Input: part model. Units: mm. Frame: model coordinates. A direction names the side the tool comes from. Round coordinates to 2 decimals unless told otherwise and drop trailing zeros. Loops run counter-clockwise (first coordinate to the right, second up) from the corner with the lowest first, then second, coordinate; pieces in that order, holes last.
1) Section A-A, the plane y = 0. Return loops of the section in (x, z).
2) Section C-C, the plane x = 4. Return loops of the section in (y, z), and give its area (3 significant figures).
3) Section B-B, the plane z = -10.5. Return loops of the section in (x, y), and give its area (3 significant figures).
4) First-contact query: pin 1 (4.5 mm diameter, centred on y = -22, z = 0.03, fed in from -X); pin 2 (4 mm diameter, centred on y = -11.03, z = -19.04, fed in from -X); pin 3 (2 mm diameter, centred on y = -1, z = 14.5, fed in from +X). Flat tips, straight axial feed; report the tip coordinate or a pass-through.
5) Access query for faces 5 (the face through (22, 4, 14)), 6 (the face through (32.5, 0, -14)), 7 (the face through (7.5, 15, -7)). Directions: +Z, -Z, +X, -X, +Y, -Y. A direction counts if a zero-diameter tool reaches every point of the face in a straight line with its end or side. Return the directions, or none.
6) Ray query, line 1 along Y through (x, z) = (22, 0.5); line 2 along X through (y, z) = (26, -3); line 3 along Z through (x, y) = (16.5, 22). Return the intervals inside material, ascending.
7) Draft query along Z for faces 1 (the face through (-0.11, 15.5, -4.88)), 2 (the face through (-7.5, 8, -10)), 3 (the face through (21.52, -10.9, -18.63)), 4 (the face through (13.99, 10.92, 16.58)). Return one class per face: pulls with the +Z half, pulls with the -Z half, needs draft (parallel to the pull), parting line crosses it, or undercut.
8) Section D-D, the plane z = 25. Return loops of the section in (x, y), and give its area (3 significant figures).
Autodesk Inventor part; units mm, degrees
ref_plane "YZ Plane" through (0, 0, 0) normal (1, 0, 0) x (0, 1, 0)
ref_plane "XZ Plane" through (0, 0, 0) normal (0, 1, 0) x (-1, 0, 0)
ref_plane "XY Plane" through (0, 0, 0) normal (0, 0, 1) x (1, 0, 0)
sketch "Skizze1" plane through (0, 0, 0) normal (1, 0, 0) x (0, 1, 0)
  circle A0 centre (0, 0) radius 12.5
  circle A1 centre (0, 0) radius 16.25
  dimension "d0" = 25
  dimension "d1" = 32.5
extrude "Extrusion1" add sketch "Skizze1" along normal mid plane 15
sketch "Skizze2" plane through (7.5, 0, 0) normal (1, 0, 0) x (0, 0, -1)
  circle A0 centre (0, 0) radius 32.5
  dimension "d5" = 65
extrude "Extrusion2" add sketch "Skizze2" along normal blind 25
sketch "Skizze4" plane through (32.5, 0, 0) normal (1, 0, 0) x (0, 0, -1)
  circle A0 centre (0, 0) radius 12.5
  dimension "d8" = 25
extrude "Extrusion3" cut sketch "Skizze4" against normal blind 30
sketch "Skizze5" plane through (7.5, 0, 0) normal (-1, 0, 0) x (0, 0, 1)
  point P0 (0, 0)
  point P1 (0.0333, -22)
  point P2 (19.0692, -10.9712)
  point P3 (19.0359, 11.0288)
  point P4 (-0.0333, 22)
  point P5 (-19.0692, 10.9712)
  point P6 (-19.0359, -11.0288)
  dimension "d18" = 22
  dimension "d21" = 360
hole "Bohrung1" at (7.5, -22, 0.0333) at (7.5, -10.9712, 19.0692) at (7.5, 11.0288, 19.0359) at (7.5, 22, -0.0333) at (7.5, 10.9712, -19.0692) at (7.5, -11.0288, -19.0359) direction (1, 0, 0) diameter 4.917 depth 12.8 tip angle 118
sketch "Skizze6" plane through (32.5, 0, 0) normal (1, 0, 0) x (0, 0, -1)
  line L0 (-16, -4) -> (-9, -4)
  line L1 (-9, -4) -> (-9, 4)
  line L2 (-9, 4) -> (-16, 4)
  line L3 (-16, 4) -> (-16, -4)
  circle A0 centre (0, 0) radius 12.5
  line L4 (-16, -4) -> (-9, 4) construction
  line L5 (-9, -4) -> (-16, 4) construction
  point P0 (-12.5, 0)
  point P1 (-11.8427, -4)
  point P2 (-11.8427, 4)
  dimension "d23" = 7
  dimension "d24" = 8
  dimension "d25" = 9
extrude "Extrusion4" cut sketch "Skizze6" against normal blind 22 contours L3 L2 A0 L0
properties part number "Befestigung bremsscheibe"
Final values:
1. outline: (-7.5, -16.25) - (7.5, -16.25) - (7.5, -32.5) - (32.5, -32.5) - (32.5, -12.5) - (-7.5, -12.5) - close; (-7.5, 12.5) - (10.5, 12.5) - (10.5, 16) - (32.5, 16) - (32.5, 32.5) - (7.5, 32.5) - (7.5, 16.25) - (-7.5, 16.25) - close
2. outline: circle Ø32.5 at (0, 0); hole circle Ø25 at (0, 0)
2. area: 339 mm2
3. outline: (-7.5, -12.4) - (7.5, -12.4) - (7.5, -30.76) - (32.5, -30.76) - (32.5, -6.78) - (-7.5, -6.78) - close; (-7.5, 6.78) - (32.5, 6.78) - (32.5, 30.76) - (7.5, 30.76) - (7.5, 12.4) - (-7.5, 12.4) - close
3. area: 1,370 mm2
4. pin 1: stops at x = 20.42
4. pin 2: stops at x = 20.57
4. pin 3: stops at x = 10.5
5. face 5: +X
5. face 6: +Z, -Z, +X, +Y, -Y
5. face 7: -X
6. line 1: y = -32.5 to -12.49, 12.49 to 32.5
6. line 2: x = 7.5 to 32.5
6. line 3: z = -23.92 to -2.49, 2.43 to 23.92
7. face 1: parting line crosses it
7. face 2: needs draft
7. face 3: undercut
7. face 4: undercut
8. outline: (7.5, -20.77) - (32.5, -20.77) - (32.5, 20.77) - (7.5, 20.77) - close
8. area: 1,040 mm2
